Geometry check sheet. Reference: the model listing, model coordinates, mm. Face numbers are marked on the shaded views. Give positions to 0.01 mm unless a question says otherwise; leave off trailing zeros. Order: outer loops, then holes, each group sorted by start corner. A loop starts at its lowest first (then second) coordinate and runs counter-clockwise, first axis right, second up. Notation, with made-up numbers: M 19,73.5 L 26,73.5 A19 cw 26,79.5 Z; hole C -32,69.5 d8. An arc over 180 degrees is marked long. Put each result on its own line as item: value. Start each with the question number.
Q1. Section check B-B on z = 33. Record the cut outline in (x, y).
Q2. Mould release check, pull along X, two halves, no side actions. Record for the marked faces 1, 2 and 3: +X half, -X half, draft (parallel to the pull), parting line (faces both ways), or undercut.
Q3. Material ranges on L1, parallel to X at y = 5, z = 33.25; L2, parallel to Z at x = 7.5, y = 5.25; L3, parallel to Z at x = 3, y = 4.5, recorded low to high.
Q4. Go/stop test with flat-tipped pins: pin 1 (1.2 mm diameter, centred on x = 4, y = 5.5, fed in from +Z); pin 2 (2 mm diameter, centred on y = 8.5, z = 31.5, fed in from -X). Record where each tip stops, or that it passes through.
Q5. Section check D-D on y = 9. Record the cut outline in (x, z), then the cut area to 3 significant figures.
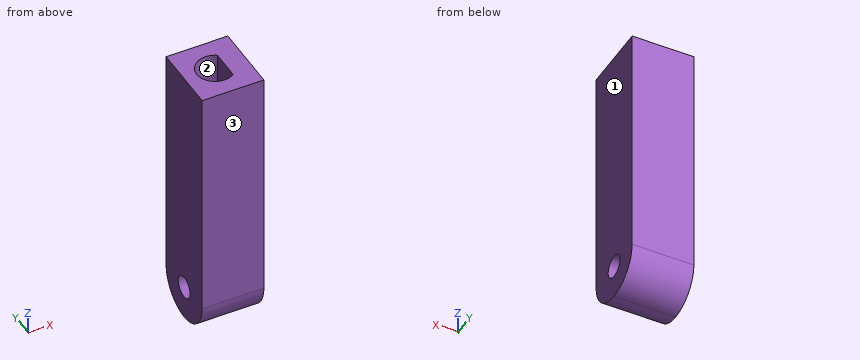
```python
from build123d import *

# Parameters (mm, degrees)
SKIZZE1_W                       = 9
SKIZZE1_H                       = 10
AUFSATZ_LINEAR_AUSTRAGEN1_DEPTH = 40
SKIZZE3_R                       = 1.65
SCHNITT_LINEAR_AUSTRAGEN2_DEPTH = 43.201895692
VERRUNDUNG1_R                   = 5
SCHNITT_LINEAR_AUSTRAGEN3_DEPTH = 10


with BuildPart() as part:
    # Skizze1 → Aufsatz-Linear austragen1 (new body)
    with BuildSketch(Plane.XY):
        with Locations((4.5, 5)):
            Rectangle(SKIZZE1_W, SKIZZE1_H)
    extrude(amount=AUFSATZ_LINEAR_AUSTRAGEN1_DEPTH)

    # Skizze3 → Schnitt-Linear austragen2 (cut, through all)
    with BuildSketch(Plane.ZY):
        with Locations((5, 5)):
            Circle(SKIZZE3_R)
    extrude(amount=-SCHNITT_LINEAR_AUSTRAGEN2_DEPTH, mode=Mode.SUBTRACT)

    # Verrundung1
    verrundung1_edges = [part.edges().sort_by_distance(p)[0] for p in [
        (4.5, 0, 0),
        (4.5, 10, 0),
    ]]
    fillet(verrundung1_edges, radius=VERRUNDUNG1_R - 0.0001)  # a hair under: the kernel refuses the full size

    # Skizze4 → Schnitt-Linear austragen3 (cut)
    with BuildSketch(Plane.XY.offset(40)):
        with BuildLine():
            Line((6, 2.815394773), (6, 7.184605227))
            ThreePointArc((6, 7.184605227), (1.85, 5), (6, 2.815394773))
        make_face()
    extrude(amount=-SCHNITT_LINEAR_AUSTRAGEN3_DEPTH, mode=Mode.SUBTRACT)


solid = part.part
```
Results found:
1. outline: M 0,0 L 9,0 L 9,10 L 0,10 Z; hole M 6,2.82 L 6,7.18 A2.65 ccw long Z
2. face 1: +X half
2. face 2: undercut
2. face 3: draft
3. L1: x = 0 to 1.85, 6 to 9
3. L2: z = 0.01 to 3.37, 6.63 to 40
3. L3: z = 0.03 to 3.43, 6.57 to 30
4. pin 1: stops at z = 30
4. pin 2: stops at x = 0
5. outline: M 0,2 L 9,2 L 9,40 L 0,40 Z
5. area: 342 mm^2
